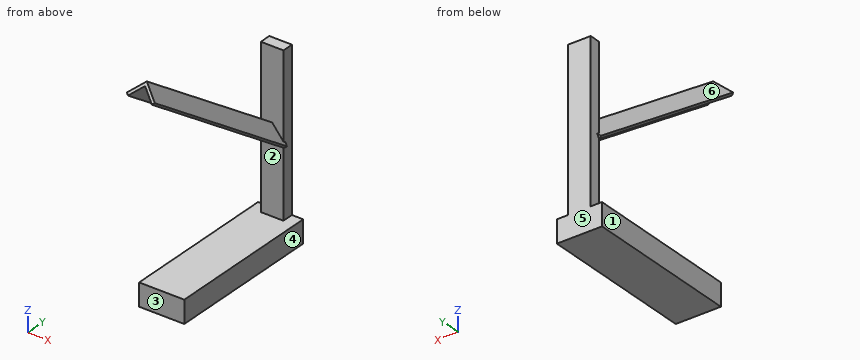
```python
from build123d import *

# Parameters (mm, degrees)
F0_W     = 50.8
F0_H     = 177.8
F1_DEPTH = 25.4
F3_W     = 25.4
F3_H     = 12.7
F4_DEPTH = 101.6
F8_DEPTH = 241.3


with BuildPart() as f1:
    # F0 (on Top) → F1 (new body)
    with BuildSketch(Plane.XY):
        with Locations((0, -76.2)):
            Rectangle(F0_W, F0_H)
    extrude(amount=-F1_DEPTH)

    # F3 (on offset) → F4 (join, symmetric)
    with BuildSketch(Plane.XY.offset(76.2)):
        with Locations((0, 6.35)):
            Rectangle(F3_W, F3_H)
    extrude(amount=F4_DEPTH, both=True)

    # F7 (on face) → F8 (join)
    with BuildSketch(Plane(origin=(0, -35.802289, 25.069033), x_dir=(-1, 0, 0), z_dir=(0, 0.819152, -0.573576))):
        Polygon((-13.470384, 62.419386), (0, 75.88977), (13.470384, 62.419386), (15.715448, 64.66445), (0, 80.379898), (-15.715448, 64.66445), align=None)
    extrude(amount=-F8_DEPTH)


solid = f1.part
```
Build history of the part. All positions in model axes, mm. Face numbers are marked on the shaded views. A direction names the side the tool comes from. Give positions to 0.01 mm unless a question says otherwise; leave off trailing zeros. Loops run counter-clockwise (first coordinate to the right, second up) from the corner with the lowest first, then second, coordinate; pieces in that order, holes last.
Item 1: Flat gauge pins, fed straight in: pin 1 (1.5 mm diameter, centred on x = 1.5, z = 30, fed in from -Y); pin 2 (14 mm diameter, centred on x = -4.5, y = 4.5, fed in from +Z); pin 3 (6.5 mm diameter, centred on y = 4, z = 90, fed in from -X). Where does each tip first touch, or does it go through?
Answers follow:
pin 1: stops at y = 0
pin 2: stops at z = 177.8
pin 3: stops at x = -12.7
Item 2: Drill centre lines: line 1 (Z direction, x = 16, y = -54); line 2 (Z direction, x = 6, y = -61); line 3 (Y direction, x = -9.5, z = 56). Where is each one in solid material? Low to high.
Answers follow:
line 1: z = -25.4 to 0
line 2: z = -25.4 to 0, 128.03 to 133.51
line 3: y = 0 to 12.7
Item 3: Slice it at A-A, the plane y = -17. List the corners of the cut face in (x, z).
Answers follow:
outline: (-25.4, -25.4) - (25.4, -25.4) - (25.4, 0) - (-25.4, 0) - close; (-15.72, 90.84) - (-13.47, 88.1) - (0, 104.55) - (13.47, 88.1) - (15.72, 90.84) - (0, 110.03) - close
Item 4: Slice it at B-B, the plane z = 199. List the corners of the cut face in (x, y).
Answers follow:
outline: (-15.72, -171.46) - (-13.47, -175.38) - (0, -151.89) - (13.47, -175.38) - (15.72, -171.46) - (0, -144.06) - close
Item 5: Pull direction Y, two halves, no side cores. Call the marked faces 4, 5 and 6: released by +Y, released by -Y, zero draft, split by the parting line, or undercut.
Answers follow:
face 4: zero draft
face 5: released by +Y
face 6: undercut
Item 6: Slice it at C-C, the plane x = 4.5. List the corners of the cut face in (y, z), and give its area (3 significant figures).
Answers follow:
outline: (-192.52, 221.95) - (0, 87.15) - (0, 0) - (-165.1, 0) - (-165.1, -25.4) - (12.7, -25.4) - (12.7, 177.8) - (0, 177.8) - (0, 92.63) - (-189.94, 225.63) - close
area: 7,820 mm2
Item 7: Which spindle directions (+Z, -Z, +X, -X, +Y, -Y) get a long thin tool onto all of the face, cutting with end or side? Do the marked faces 1, 2 and 3. Say none if no direction does.
Answers follow:
face 1: +Z, -Z, -X, +Y, -Y
face 2: -Y
face 3: -Z, +X, -X, -Y
Item 8: Slice it at D-D, the plane y = -171. List the corners of the cut face in (x, z).
Answers follow:
outline: (-15.72, 198.68) - (-13.47, 195.94) - (0, 212.38) - (13.47, 195.94) - (15.72, 198.68) - (0, 217.86) - close
